```python
from build123d import *

# Parameters (mm, degrees)
SKETCH1_R           = 8.7
BOSS_EXTRUDE1_DEPTH = 2.3
SKETCH2_R           = 6
BOSS_EXTRUDE2_DEPTH = 1.25
SKETCH3_R           = 7.4
SKETCH3_R_2         = 4.1
SKETCH3_R_3         = 3.2
CUT_EXTRUDE2_DEPTH  = 1.5
BOSS_EXTRUDE3_START = 1.3
SKETCH6_R           = 3.2
BOSS_EXTRUDE3_DEPTH = 1.3
SKETCH7_R           = 2.3
CUT_EXTRUDE3_DEPTH  = 13.751568531
SKETCH9_R           = 0.75
CUT_EXTRUDE4_DEPTH  = 0.2
CIRPATTERN1_COUNT   = 6
BOSS_EXTRUDE4_DEPTH = 1.5
CIRPATTERN2_COUNT   = 6
FILLET2_R           = 0.2


with BuildPart() as part:
    # Sketch1 → Boss-Extrude1 (new body)
    with BuildSketch(Plane(origin=(0, 0, 0), x_dir=(1, 0, 0), z_dir=(0, 1, 0))):
        with Locations(Location((0, 0, 0), (0, 0, 270))):
            Circle(SKETCH1_R)
    extrude(amount=BOSS_EXTRUDE1_DEPTH)

    # Sketch2 → Boss-Extrude2 (add)
    with BuildSketch(Plane(origin=(0, 2.3, 0), x_dir=(1, 0, 0), z_dir=(0, 1, 0))):
        with Locations(Location((0, 0, 0), (0, 0, 270))):
            Circle(SKETCH2_R)
    extrude(amount=BOSS_EXTRUDE2_DEPTH)

    # Sketch3 → Cut-Extrude2 (cut)
    # profile 1 of 2: a face of its own
    with BuildSketch(Plane.XZ):
        with Locations(Location((0, 0, 0), (0, 0, 270))):
            Circle(SKETCH3_R)
        with Locations(Location((0, 0, 0), (0, 0, 270))):
            Circle(SKETCH3_R_2, mode=Mode.SUBTRACT)
    # profile 2 of 2: a face of its own
    with BuildSketch(Plane.XZ):
        with Locations(Location((0, 0, 0), (0, 0, 270))):
            Circle(SKETCH3_R_3)
    extrude(amount=-CUT_EXTRUDE2_DEPTH, mode=Mode.SUBTRACT)

    # Sketch6 → Boss-Extrude3 (add)
    with BuildSketch(Plane.XZ.offset(-1.5).offset(BOSS_EXTRUDE3_START)):
        with Locations(Location((0, 0, 0), (0, 0, 270))):
            Circle(SKETCH6_R)
    extrude(amount=-BOSS_EXTRUDE3_DEPTH)

    # Sketch7 → Cut-Extrude3 (cut, through all)
    with BuildSketch(Plane.XZ.offset(-0.2)):
        with Locations(Location((0, 0, 0), (0, 0, 270))):
            Circle(SKETCH7_R)
    extrude(amount=-CUT_EXTRUDE3_DEPTH, mode=Mode.SUBTRACT)

    # Mirror4: part across plane


with BuildPart() as part_1:
    add(part.part)
    add(part.part.mirror(Plane.ZX.offset(3.55)))

    # Sketch9 → Cut-Extrude4 (cut)
    with BuildSketch(Plane.XZ.offset(-1.5)):
        with Locations(Location((0, -5.557983599, 0), (0, 0, 270))):
            Circle(SKETCH9_R)
    cut_extrude4 = extrude(amount=-CUT_EXTRUDE4_DEPTH, mode=Mode.SUBTRACT)

    # CirPattern1: Cut-Extrude4 ×6 about axis
    cirpattern1_axis = Axis((0, 0, 0), (0, 1, 0))
    for i in range(1, CIRPATTERN1_COUNT):
        add(cut_extrude4.rotate(cirpattern1_axis, i * 360 / CIRPATTERN1_COUNT), mode=Mode.SUBTRACT)

    # Sketch10 → Boss-Extrude4 (add)
    with BuildSketch(Plane(origin=(0, 7.1, 0), x_dir=(1, 0, 0), z_dir=(0, 1, 0))):
        with BuildLine():
            Line((7.321025788, -1.078230685), (4.042247415, -0.68573744))
            ThreePointArc((4.042247415, -0.68573744), (4.003777056, -0.883045462), (3.955681811, -1.078230685))
            Line((3.955681811, -1.078230685), (7.25195199, -1.472817823))
            ThreePointArc((7.25195199, -1.472817823), (7.289159422, -1.275991739), (7.321025788, -1.078230685))
        make_face()
        with BuildLine():
            Line((7.368334518, -0.683846791), (4.092875821, 0.241593702))
            ThreePointArc((4.092875821, 0.241593702), (4.074467049, 0.456856947), (4.044744505, 0.670851615))
            Line((4.044744505, 0.670851615), (7.394863003, -0.275683086))
            ThreePointArc((7.394863003, -0.275683086), (7.384419386, -0.479948264), (7.368334518, -0.683846791))
        make_face()
    boss_extrude4 = extrude(amount=-BOSS_EXTRUDE4_DEPTH)

    # CirPattern2: Boss-Extrude4 ×6 about axis
    cirpattern2_axis = Axis((0, 0, 0), (0, 1, 0))
    for i in range(1, CIRPATTERN2_COUNT):
        add(boss_extrude4.rotate(cirpattern2_axis, i * 360 / CIRPATTERN2_COUNT))

    # Fillet2
    fillet2_edges = [part_1.edges().sort_by_distance(p)[0] for p in [
        (2.603346793, 6.35, 3.167425686),
        (2.255664194, 6.35, 3.423737584),
        (1.427257664, 6.35, 3.84355767),
        (1.044065742, 6.35, 3.96483628),
        (-1.441397712, 6.35, 3.838277301),
        (-1.837211627, 6.35, 3.665331286),
        (-2.614989751, 6.35, 3.157820229),
        (-2.91161607, 6.35, 2.886605595),
        (-4.044744505, 6.35, 0.670851615),
        (-4.092875821, 6.35, 0.241593702),
        (-4.042247415, 6.35, -0.68573744),
        (-3.955681811, 6.35, -1.078230685),
        (-2.603346793, 6.35, -3.167425686),
        (-2.255664194, 6.35, -3.423737584),
        (-1.427257664, 6.35, -3.84355767),
        (-1.044065742, 6.35, -3.96483628),
        (1.441397712, 6.35, -3.838277301),
        (1.837211627, 6.35, -3.665331286),
        (2.614989751, 6.35, -3.157820229),
        (2.91161607, 6.35, -2.886605595),
        (4.044744505, 6.35, -0.670851615),
        (4.092875821, 6.35, -0.241593702),
        (4.042247415, 6.35, 0.68573744),
        (3.955681811, 6.35, 1.078230685),
    ]]
    fillet(fillet2_edges, radius=FILLET2_R)


solid = part_1.part
```
Work out the finished part from the listing and answer in its coordinate system (mm). A direction names the side the tool comes from. Give positions to 0.01 mm unless a question says otherwise; leave off trailing zeros. Order: outer loops, then holes, each group sorted by start corner. A loop starts at its lowest first (then second) coordinate and runs counter-clockwise, first axis right, second up. Notation, with made-up numbers: (0.25, -10) -> (25.25, -10) arc R37 cw to (25.25, 28) -> close; hole circle Ø4 at (78, -1). An arc over 180 degrees is marked (long way). Answer as CSV lines item,"result". Start each with the question number.
(1) Section B-B, the plane y = 6.25 is taken. Give the number of separate pieces and of enclosed holes in the cut face, plus the area to 3 significant figures.
(2) Section A-A, the plane x = -7 is taken. Write down the section's boundary in (y, z).
(3) Consider line 1 along Y through (x, z) = (5.25, -4.5); line 2 along Z through (x, y) = (-0.5, 1.25) (3 decimals); line 3 along X through (y, z) = (1.25, 1.25). Determine where each line is inside the solid, lowest interval first.
(4) Which of the six approach directions +Z, -Z, +X, -X, +Y, -Y give full straight-line access (tool end or side, diameter ignored) to faces 1 (the cylindrical face through (4.065, 0.74, 0.534)), 2 (the flat face through (3.17, 6.36, -4.96)), 3 (the cylindrical face through (0.691, 3.597, -2.194))?
(5) Each of these flat-tipped pins is pushed along its axis until it touches: pin 1 Ø1.6 at (x, z) = (4.5, -2.5) entering from -Y; pin 2 Ø2 at (x, z) = (4.81, 2.78) entering from +Y; pin 3 Ø3 at (y, z) = (3, -3) entering from -X. Where does it stop, or does it pass through?
(6) For a pull along Z with two mould halves and no side action, classify faces 4 (the cylindrical face through (-5.3, 1.1, -6.9)), 5 (the flat face through (-5.666, 6.36, -1.283)), 6 (the flat face through (1, 5.6, -6)) as released by +Z, released by -Z, zero draft, split by the parting line, or undercut.
Entries:
1,separate pieces,"1"
1,enclosed holes,"13"
1,area,"118 mm²"
2,outline,"(0, -5.17) -> (2.3, -5.17) -> (2.3, 5.17) -> (0, 5.17) -> (0, 2.4) -> (1.5, 2.4) -> (1.5, -2.4) -> (0, -2.4) -> close; (4.8, -5.17) -> (7.1, -5.17) -> (7.1, -2.4) -> (5.6, -2.4) -> (5.6, -1.44) -> (7.1, -1.44) -> (7.1, -1.04) -> (5.6, -1.04) -> (5.6, -0.58) -> (7.1, -0.58) -> (7.1, -0.16) -> (5.6, -0.16) -> (5.6, 2.4) -> (7.1, 2.4) -> (7.1, 5.17) -> (4.8, 5.17) -> close"
3,line 1,"1.5 to 2.3, 4.8 to 5.6"
3,line 2,"-8.686 to -7.383, -4.069 to -2.245, 2.245 to 4.069, 7.383 to 8.686"
3,line 3,"-8.61 to -7.29, -3.9 to -1.93, 1.93 to 3.9, 7.29 to 8.61"
4,face 1,"-Y"
4,face 2,"+Y"
4,face 3,"+Y, -Y"
5,pin 1,"y = 1.5"
5,pin 2,"y = 5.6"
5,pin 3,"x = -8.54"
6,face 4,"split by the parting line"
6,face 5,"undercut"
6,face 6,"undercut"
